from build123d import *

# Parameters (mm, degrees)
BOSS_EXTRUDE1_DEPTH = 15
CUT_EXTRUDE1_DEPTH  = 172.190683158
BOSS_EXTRUDE2_START = 3.1
SKETCH4_R           = 2.55
BOSS_EXTRUDE2_DEPTH = 5.8


with BuildPart() as part:
    # Sketch1 → Boss-Extrude1 (new, symmetric)
    with BuildSketch(Plane.XY):
        with BuildLine():
            Line((-60, 0), (60, 0))
            ThreePointArc((60, 0), (14.978542663, 64.137960841), (15, 142.5))
            Line((15, 142.5), (15, 157.5))
            ThreePointArc((15, 157.5), (-32.469836355, 83.497541122), (-60, 0))
        make_face()
    extrude(amount=BOSS_EXTRUDE1_DEPTH, both=True)

    # Sketch3 → Cut-Extrude1 (cut, through all)
    with BuildSketch(Plane.XY.offset(15)):
        with BuildLine():
            Line((10, 143.26466224), (10, 143.272073771))
            ThreePointArc((10, 143.272073771), (-29.664180918, 77.705142353), (-53.876409624, 5))
            Line((-53.876409624, 5), (46.39672745, 5))
            ThreePointArc((46.39672745, 5), (8.391850624, 68.918473527), (10, 143.26466224))
        make_face()
    extrude(amount=-CUT_EXTRUDE1_DEPTH, mode=Mode.SUBTRACT)

    # Sketch4 → Boss-Extrude2 (add)
    with BuildSketch(Plane.XY.offset(BOSS_EXTRUDE2_START)):
        with BuildLine():
            Line((25, 145.5), (20.196152423, 145.5))
            Line((20.196152423, 145.5), (15, 142.5))
            Line((15, 142.5), (15, 157.5))
            Line((15, 157.5), (20.196152423, 154.5))
            Line((20.196152423, 154.5), (25, 154.5))
            ThreePointArc((25, 154.5), (29.5, 150), (25, 145.5))
        make_face()
        with Locations((25, 150)):
            Circle(SKETCH4_R, mode=Mode.SUBTRACT)
    boss_extrude2 = extrude(amount=BOSS_EXTRUDE2_DEPTH)

    # Mirror1: Boss-Extrude2 across plane
    add(boss_extrude2.mirror(Plane.XY))


solid = part.part
Input: part model. Units: mm. Frame: model coordinates. A direction names the side the tool comes from. Coordinates: 2 decimals unless noted, no trailing zeros. Write each loop counter-clockwise with the first axis right and the second up, starting at its lowest first coordinate (ties: lowest second). Pieces come first, ordered by that corner, then holes. Notation, with made-up numbers: M -19,62.5 L 22,62.5 A16 ccw 22,87.5 Z; hole C 71,42 d3. An arc over 180 degrees is marked long. Answer as a JSON object with one key per item and string values. Group by question number.
(1) Mould query, pull axis X, two halves, no side actions, for faces 1 (the face through (-29.21, 78.68, 0.21)), 2 (the face through (21, 150, -3.1)), 3 (the face through (17.6, 156, 6)), 4 (the face through (24.67, 152.53, -5.96)). Classes: pulls with the +X half, pulls with the -X half, needs draft (parallel to the pull), parting line crosses it, or undercut.
(2) Set-up query: faces 5 (the face through (15, 150, 12)), 6 (the face through (15, 150, 0)), 7 (the face through (17.6, 144, 6)), 8 (the face through (-4, 5, 0)), 9 (the face through (15, 150, -12)). Return all of +Z, -Z, +X, -X, +Y, -Y with unobstructed straight access to the full face (end or side cutting, diameter ignored); none if empty.
(3) Ray query, line 1 along X through (y, z) = (150, 5.3); line 2 along Y through (x, z) = (25, -6.1); line 3 along Y through (x, z) = (26.5, -5). Return the intervals inside material, ascending. Write a range as [from, to].
(4) Section C-C on y = 132.5. Output: boundary loops of the cut face in (x, z), plus the area to 3 significant figures.
(5) Contact query for flat-ended pins moving along their axis: P1, Ø2.5, axis at x = 23.5, z = 6, coming from the +Y side; P2, Ø4.5, axis at x = 25.5, y = 148.5, coming from the -Z side; P3, Ø10, axis at y = 111.5, z = -4.5, coming from the -X side. Output: stop coordinate, or through.
(6) Section B-B on x = -11.5. Output: boundary loops of the cut face in (y, z), plus the area to 3 significant figures.
(7) Section A-A on y = 150. Output: boundary loops of the cut face in (x, z), plus the area to 3 significant figures.
Result set:
{
 "1": {"face 1": "undercut", "face 2": "needs draft", "face 3": "pulls with the +X half", "face 4": "undercut"},
 "2": {"face 5": "+Z, +X, +Y", "face 6": "+X, +Y", "face 7": "+Z, -Z, +X", "face 8": "+Z, -Z", "face 9": "-Z, +X, +Y"},
 "3": {"line 1": "x = [8.9, 22.45], [27.55, 29.5]", "line 2": "y = [0, 5], [30.89, 40.7], [145.5, 147.45], [152.55, 154.5]", "line 3": "y = [0, 5], [28.58, 38.04], [145.76, 147.94], [152.06, 154.24]"},
 "4": {"outline": "M -4.06,-15 L 2.05,-15 L 2.05,15 L -4.06,15 Z; M 7.14,-15 L 12.27,-15 L 12.27,15 L 7.14,15 Z", "area": "337 mm2"},
 "5": {"P1": "stops at y = 154.5", "P2": "stops at z = -8.9", "P3": "stops at x = -20.45"},
 "6": {"outline": "M 0,-15 L 5,-15 L 5,15 L 0,15 Z; M 111.85,-15 L 121.32,-15 L 121.32,15 L 111.85,15 Z", "area": "434 mm2"},
 "7": {"outline": "M 8.9,-15 L 15,-15 L 15,-8.9 L 22.45,-8.9 L 22.45,-3.1 L 15,-3.1 L 15,3.1 L 22.45,3.1 L 22.45,8.9 L 15,8.9 L 15,15 L 8.9,15 Z; M 27.55,-8.9 L 29.5,-8.9 L 29.5,-3.1 L 27.55,-3.1 Z; M 27.55,3.1 L 29.5,3.1 L 29.5,8.9 L 27.55,8.9 Z", "area": "292 mm2"}
}
